Autodesk Inventor part; units mm, degrees
ref_plane "Work Plane1" through (0, 11.5, 0) normal (0, 1, 0) x (1, 0, 0)
ref_plane "Work Plane2" through (0, 22, 0) normal (0, 1, 0) x (1, 0, 0)
ref_plane "YZ Plane" through (0, 0, 0) normal (1, 0, 0) x (0, 1, 0)
sketch "Sketch1" plane through (0, 0, 0) normal (0, 1, 0) x (-1, 0, 0)
  circle A0 centre (0, 0) radius 2.9
  circle A1 centre (0, 0) radius 1.6
  dimension "d0" = 3.2
  dimension "d1" = 5.8
extrude "Extrusion1" add sketch "Sketch1" along normal blind 23
ref_plane "Work Plane1" through (0, 11.5, 0) normal (0, 1, 0) x (1, 0, 0)
sketch "Sketch3" plane through (0, 11.5, 0) normal (0, 1, 0) x (1, 0, 0)
  circle A0 centre (0, 0) radius 1.6 construction
  circle A1 centre (0, 0) radius 2.2
  circle A2 centre (0, 0) radius 2.9
  dimension "d12" = 0.7
extrude "Extrusion3" cut sketch "Sketch3" along normal mid plane 0.5
ref_plane "Work Plane2" through (0, 22, 0) normal (0, 1, 0) x (1, 0, 0)
sketch "Sketch4" plane through (0, 22, 0) normal (0, 1, 0) x (1, 0, 0)
  circle A0 centre (0, 0) radius 2.9
  circle A1 centre (0, 0) radius 2.2
  dimension "d9" = 0.7
extrude "Extrusion4" cut sketch "Sketch4" along normal mid plane 0.5
mirror "Mirror1" about plane through (0, 11.5, 0) normal (0, 1, 0) of "Extrusion4"
properties part number "fullbar"
Build history of the part. All positions in model axes, mm. A direction names the side the tool comes from. Give positions to 0.01 mm unless a question says otherwise; leave off trailing zeros. Order: outer loops, then holes, each group sorted by start corner. A loop starts at its lowest first (then second) coordinate and runs counter-clockwise, first axis right, second up. Notation, with made-up numbers: M -21,69.5 L 17,69.5 A22 ccw 17,92.5 Z; hole C -35,8 d11. An arc over 180 degrees is marked long. Use one line per item in the form item = value.
1) Two-plate mould, pull along Y, no slides. Class faces 3 (the face through (-1.25, 0, -1.25)), 4 (the face through (0.9, 0.75, -2.2)), 5 (the face through (-1.25, 23, -1.25)), 6 (the face through (-0.9, 21.75, -2.2)): released by +Y, released by -Y, zero draft, split by the parting line, or undercut.
Calculated:
face_3 = released by -Y
face_4 = undercut
face_5 = released by +Y
face_6 = undercut
2) Drop flat-ended pins along their axis: pin 1 (1.5 mm diameter, centred on y = 4.5, z = 1, fed in from -X); pin 2 (1 mm diameter, centred on x = -2, y = 11.5, fed in from +Z). Give the stop position or say it passes through.
Calculated:
pin_1 = -2.89
pin_2 = 2.44
3) Probe probe 1 along Y at (x, z) = (-2.4, -0.5); probe 2 along Z at (x, y) = (0, 10.75); probe 3 along X at (y, z) = (10, 1.35). List the from-to ranges inside material, lowest first.
Calculated:
probe_1 = 0 to 0.75, 1.25 to 11.25, 11.75 to 21.75, 22.25 to 23
probe_2 = -2.9 to -1.6, 1.6 to 2.9
probe_3 = -2.57 to -0.86, 0.86 to 2.57
4) Saw through at C-C (y = 12.25). Give the cut face in (x, z).
Calculated:
outline = C 0,0 d5.8; hole C 0,0 d3.2
5) Saw through at D-D (z = 1.9). Give the cut face in (x, y), plus the area to 3 significant figures.
Calculated:
outline = M -2.19,0 L 2.19,0 L 2.19,0.75 L 1.11,0.75 L 1.11,1.25 L 2.19,1.25 L 2.19,11.25 L 1.11,11.25 L 1.11,11.75 L 2.19,11.75 L 2.19,21.75 L 1.11,21.75 L 1.11,22.25 L 2.19,22.25 L 2.19,23 L -2.19,23 L -2.19,22.25 L -1.11,22.25 L -1.11,21.75 L -2.19,21.75 L -2.19,11.75 L -1.11,11.75 L -1.11,11.25 L -2.19,11.25 L -2.19,1.25 L -1.11,1.25 L -1.11,0.75 L -2.19,0.75 Z
area = 97.5 mm2
6) Tool access for faces 1 (the face through (1.27, 11.34, 0.97)), 2 (the face through (-0.9, 11.75, -2.2)): list every direction of +Z, -Z, +X, -X, +Y, -Y with a clear straight run to the whole face (end or side of a thin tool).
Calculated:
face_1 = +Y, -Y
face_2 = none
